from build123d import *

# Parameters (mm, degrees)
F0_R     = 10
F1_DEPTH = 14
F0_R_2   = 3.5
F2_DEPTH = 3


with BuildPart() as f1:
    # F0 (on Front) → F1 (new body)
    with BuildSketch(Plane.XZ):
        Circle(F0_R)
        Polygon((-5.184207, 5.020691), (1.755942, 7), (6.940149, 1.979309), (5.184207, -5.020691), (-1.755942, -7), (-6.940149, -1.979309), align=None, mode=Mode.SUBTRACT)
    extrude(amount=F1_DEPTH)

    # F0 (on Front) → F2 (join)
    with BuildSketch(Plane.XZ):
        Polygon((6.940149, 1.979309), (1.755942, 7), (-5.184207, 5.020691), (-6.940149, -1.979309), (-1.755942, -7), (5.184207, -5.020691), align=None)
        Circle(F0_R_2, mode=Mode.SUBTRACT)
    extrude(amount=F2_DEPTH)


solid = f1.part
Source: CAD feature listing. Evaluate the final solid. Frame: model axes, mm. A direction names the side the tool comes from. Round coordinates to 2 decimals unless told otherwise and drop trailing zeros. Loops run counter-clockwise (first coordinate to the right, second up) from the corner with the lowest first, then second, coordinate; pieces in that order, holes last. Notation, with made-up numbers: (74.5, 24) -> (107.5, 24) arc R30 ccw to (107.5, 54) -> close; hole circle Ø5 at (49, 58.5). An arc over 180 degrees is marked (long way). Answer as a JSON object with one key per item and string values. Group by question number.
Q1. Ray query, line 1 (Z direction, x = 0, y = -1.75); line 2 (Y direction, x = 5, z = -5); line 3 (X direction, y = -3.25, z = -0.5). Return the intervals inside material, ascending. Write a range as from..to.
Q2. Section query A-A (x = 0). Output: boundary loops of the cut face in (y, z).
Q3. Access query for faces 4 (the cylindrical face through (3.233, -1.479, -1.341)), 5 (the flat face through (4.312, -8.423, 4.525)). Directions: +Z, -Z, +X, -X, +Y, -Y. A direction counts if a zero-diameter tool reaches every point of the face in a straight line with its end or side. Return the directions, or none.
Q4. Section query D-D (z = -5.75). Output: boundary loops of the cut face in (x, y).
Q5. Contact query for flat-ended pins moving along their axis: P1, Ø1, axis at y = -9.5, z = 3, coming from the -X side; P2, Ø8, axis at x = 0, z = 0, coming from the -Y side; P3, Ø5, axis at x = 7, y = -6, coming from the -Z side. Output: stop coordinate, or through.
Q6. Section query B-B (z = 0). Output: boundary loops of the cut face in (x, y).
Q7. Section query C-C (y = -9). Output: boundary loops of the cut face in (x, z), plus the area to 3 significant figures.
Q8. Mould query, pull axis X, two halves, no side actions, for faces 1 (the cylindrical face through (-2.17, -6.9, -9.76)), 2 (the flat face through (7, -14, 0)), 3 (the flat face through (6.074, -8.423, -1.472)). Classes: pulls with the +X half, pulls with the -X half, needs draft (parallel to the pull), parting line crosses it, or undercut.
Completed:
{
 "1": {"line 1": "-10..-3.5, 3.5..10", "line 2": "-3..0", "line 3": "-9.99..-6.57, 6.32..9.99"},
 "2": {"outline": "(-14, -10) -> (0, -10) -> (0, -3.5) -> (-3, -3.5) -> (-3, -6.5) -> (-14, -6.5) -> close; (-14, 6.5) -> (-3, 6.5) -> (-3, 3.5) -> (0, 3.5) -> (0, 10) -> (-14, 10) -> close"},
 "3": {"face 4": "+Y, -Y", "face 5": "-Y"},
 "4": {"outline": "(-8.18, -14) -> (-3.05, -14) -> (-3.05, -3) -> (2.63, -3) -> (2.63, -14) -> (8.18, -14) -> (8.18, 0) -> (-8.18, 0) -> close"},
 "5": {"P1": "x = -9.68", "P2": "y = -3", "P3": "z = -8.93"},
 "6": {"outline": "(-10, -14) -> (-6.44, -14) -> (-6.44, -3) -> (-3.5, -3) -> (-3.5, 0) -> (-10, 0) -> close; (3.5, -3) -> (6.44, -3) -> (6.44, -14) -> (10, -14) -> (10, 0) -> (3.5, 0) -> close"},
 "7": {"outline": "circle Ø20 at (0, 0); hole (-6.94, -1.98) -> (-1.76, -7) -> (5.18, -5.02) -> (6.94, 1.98) -> (1.76, 7) -> (-5.18, 5.02) -> close", "area": "179 mm²"},
 "8": {"face 1": "parting line crosses it", "face 2": "needs draft", "face 3": "undercut"}
}
